The listing builds one solid part. Answer for the finished solid, in the listing's coordinates (mm). Give positions to 0.01 mm unless a question says otherwise; leave off trailing zeros. Order: outer loops, then holes, each group sorted by start corner. A loop starts at its lowest first (then second) coordinate and runs counter-clockwise, first axis right, second up. Notation, with made-up numbers: (58.5, 29.5) -> (85.5, 29.5) arc R9 ccw to (85.5, 40.5) -> close; hole circle Ø11 at (0.5, 22.5). An arc over 180 degrees is marked (long way). One line per question, with ' | ' between items. Start each with the question number.
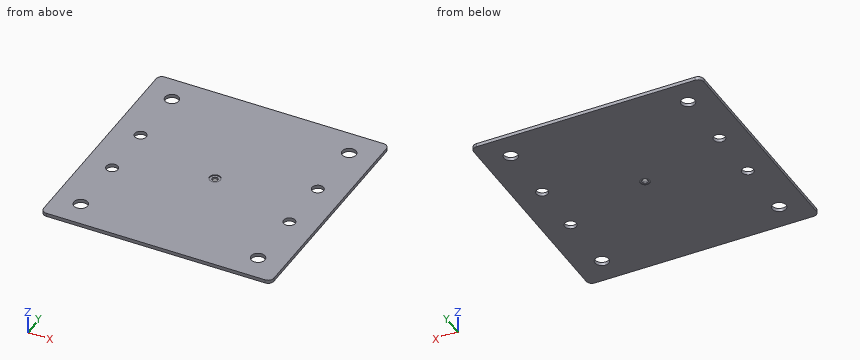
Autodesk Inventor part; units mm, degrees
ref_plane "YZ Plane" through (0, 0, 0) normal (1, 0, 0) x (0, 1, 0)
ref_plane "XZ Plane" through (0, 0, 0) normal (0, 1, 0) x (-1, 0, 0)
ref_plane "XY Plane" through (0, 0, 0) normal (0, 0, 1) x (1, 0, 0)
sketch "Sketch1" plane through (0, 0, 0) normal (0, 0, 1) x (1, 0, 0)
  line L0 (100, 100) -> (-100, 100)
  line L1 (-100, 100) -> (-100, -100)
  line L2 (-100, -100) -> (100, -100)
  line L3 (100, -100) -> (100, 100)
  line L4 (100, 100) -> (-100, -100) construction
  line L5 (-100, 100) -> (100, -100) construction
  point P0 (0, 0)
  dimension "d0" = 200
  dimension "d1" = 200
extrude "Extrusion1" add sketch "Sketch1" along normal blind 3
fillet "Fillet1" radius 5 4 edges at (100, 100, 1.5) (-100, 100, 1.5) (100, -100, 1.5) (-100, -100, 1.5)
sketch "Sketch2" plane through (0, 0, 3) normal (0, 0, 1) x (1, 0, 0)
  circle A0 centre (0, 0) radius 2.55
  dimension "d5" = 5.1
extrude "Extrusion2" cut sketch "Sketch2" against normal blind 10
sketch "Sketch3" plane through (0, 0, 3) normal (0, 0, 1) x (1, 0, 0)
  circle A0 centre (0, 0) radius 4.75
  dimension "d10" = 9.5
extrude "Extrusion3" cut sketch "Sketch3" against normal blind 0.7
sketch "Sketch4" plane through (0, 0, 0) normal (0, 0, -1) x (-1, 0, 0)
  point P0 (0, 0)
sketch "Sketch5" plane through (0, 0, 0) normal (0, 0, -1) x (-1, 0, 0)
  point P0 (0, 0)
sketch "Sketch6" plane through (0, 0, 0) normal (0, 0, -1) x (-1, 0, 0)
  circle A0 centre (-77, 77) radius 6
  line L0 (-93.7439, 99.9999) -> (-93.7439, -0.0001)
  line L1 (-93.7439, -0.0001) -> (78.7368, -0.0001)
  circle A1 centre (-77, -77.0002) radius 6
  line L2 (95, -100) -> (-95, -100)
  line L3 (0, -100) -> (0, 48.6306)
  circle A2 centre (77, 77) radius 6
  circle A3 centre (77, -77.0002) radius 6
  line L4 (-95, 100) -> (95, 100)
  line L5 (-100, -95) -> (-100, 95)
  point P0 (0, 0)
  point P1 (-93.7439, 89.8675)
  point P2 (-93.7439, 85.1564)
  dimension "d11" = 12
  dimension "d13" = 100
  dimension "d22" = 23
  dimension "d23" = 23
extrude "Extrusion4" cut sketch "Sketch6" against normal blind 10
sketch "Sketch8" plane through (0, 0, 0) normal (0, 0, -1) x (-1, 0, 0)
  circle A0 centre (0, 0) radius 4.24
  dimension "d19" = 8.48
extrude "Extrusion6" cut sketch "Sketch8" against normal blind 0.5
ref_plane "Work Plane1" through (0, 0, 1.5) normal (0, 0, -1) x (-1, 0, 0)
ref_plane "Work Plane2" through (0.0302, -1.2496, -9.3454) normal (0, 0, -1) x (0.0242, -0.9997, 0)
sketch "Sketch9" plane through (0, 0, 3) normal (0, 0, 1) x (1, 0, 0)
  line L0 (-100, -40) -> (100, -40)
  line L1 (100, -40) -> (100, 40)
  line L2 (100, 40) -> (-100, 40)
  line L3 (-100, 40) -> (-100, -40)
  circle A0 centre (0, 0) radius 2.55
  line L4 (-100, -40) -> (100, 40) construction
  line L5 (100, -40) -> (-100, 40) construction
  circle A1 centre (-77, 24) radius 5.05
  line L6 (0, 0) -> (0, 19)
  line L7 (0, 0) -> (22.4044, 0)
  circle A2 centre (77, 24) radius 5.05
  circle A3 centre (-77, -24) radius 5.05
  circle A4 centre (77, -24) radius 5.05
  dimension "d24" = 200
  dimension "d25" = 80
  dimension "d26" = 10.1
  dimension "d27" = 23
  dimension "d28" = 16
extrude "Extrusion7" cut sketch "Sketch9" against normal blind 10 contours A1 | A2 | A3 | A4
properties part number "Base" material "Aluminum 6061"
(1) The part is cut by section B-B on x = 77. Determine the outline of the cut face in (y, z), plus the area to 3 significant figures.
(2) The part is cut by section A-A on y = 77. Determine the outline of the cut face in (x, z), plus the area to 3 significant figures.
(3) Consider line 1 (X direction, y = -24.5, z = 2); line 2 (Y direction, x = -77, z = 0.7); line 3 (Y direction, x = 71.5, z = 2.25). Determine where each line is inside the solid, lowest interval first.
(4) The part is cut by section C-C on x = 0. Determine the outline of the cut face in (y, z).
(5) Given P1, Ø13, axis at x = -77, y = -24, coming from the -Z side; P2, Ø7, axis at x = 0, y = 0, coming from the +Z side; P3, Ø4, axis at x = 1, y = 0.5, coming from the -Z side, each flat-ended and moving along its own axis, determine where each tip first touches the part or whether it passes through.
Result sheet:
1) outline: (-100, 0) -> (-83, 0) -> (-83, 3) -> (-100, 3) -> close; (-71, 0) -> (-29.05, 0) -> (-29.05, 3) -> (-71, 3) -> close; (-18.95, 0) -> (18.95, 0) -> (18.95, 3) -> (-18.95, 3) -> close; (29.05, 0) -> (71, 0) -> (71, 3) -> (29.05, 3) -> close; (83, 0) -> (100, 0) -> (100, 3) -> (83, 3) -> close | area: 467 mm^2
2) outline: (-100, 0) -> (-83, 0) -> (-83, 3) -> (-100, 3) -> close; (-71, 0) -> (71, 0) -> (71, 3) -> (-71, 3) -> close; (83, 0) -> (100, 0) -> (100, 3) -> (83, 3) -> close | area: 528 mm^2
3) line 1: x = -100 to -82.03, -71.97 to 71.97, 82.03 to 100 | line 2: y = -100 to -83, -71 to -29.05, -18.95 to 18.95, 29.05 to 71, 83 to 100 | line 3: y = -100 to -79.4, -74.6 to 74.6, 79.4 to 100
4) outline: (-100, 0) -> (-4.24, 0) -> (-4.24, 0.5) -> (-2.55, 0.5) -> (-2.55, 2.3) -> (-4.75, 2.3) -> (-4.75, 3) -> (-100, 3) -> close; (2.55, 0.5) -> (4.24, 0.5) -> (4.24, 0) -> (100, 0) -> (100, 3) -> (4.75, 3) -> (4.75, 2.3) -> (2.55, 2.3) -> close
5) P1: stops at z = 0 | P2: stops at z = 2.3 | P3: stops at z = 0.5
